Could you check a few things on this model? Use its own coordinates, in mm. A direction names the side the tool comes from. Give positions to 0.01 mm unless a question says otherwise; leave off trailing zeros. Loops run counter-clockwise (first coordinate to the right, second up) from the corner with the lowest first, then second, coordinate; pieces in that order, holes last.
1. Imagine slicing it at A-A (x = -54.5). List the corners of the cut face in (y, z) for me, plus the area to 3 significant figures.
2. For faces 4 (the cylindrical face through (-2.52, -3.79, -17.07)), 5 (the cylindrical face through (-52.874, -11.923, 3.755)), 6 (the flat face through (6.801, 13, -13)), 7 (the cylindrical face through (-34.37, -29.97, 1.32)), 8 (the conical face through (-12.821, -14.747, -11.307)), which set-ups out of +Z, -Z, +X, -X, +Y, -Y let a thin tool reach every point of the face, with its end or its side?
3. Imagine slicing it at B-B (y = -26). Count the separate pieces of the cut face and the enclosed holes in it, plus the area to 3 significant figures.
4. For P1, Ø8, axis at x = -2, y = 17, coming from the -Z side; P2, Ø5, axis at x = -44, z = -15, coming from the -Y side; P3, Ø1, axis at x = -39, y = 10, coming from the -Z side, each with a flat end and sliding along its axis, tell me the tip position at first contact or that it passes through.
5. I need wall thicknesses on line 1 along X through (y, z) = (-1, 26); line 2 along X through (y, z) = (-25, -13); line 3 along X through (y, z) = (11.5, 4). Which ranges of each line are inside material? Lowest first, please.
6. Thinking about a two-plate mould opening in Z: for faces 1 (the flat face through (-12.099, 0, 0)), 2 (the flat face through (-44, 0, -13)), 3 (the cylindrical face through (-10.72, -1.32, -29.97)), which applies, +Z half, -Z half, draft (parallel to the pull), parting line (faces both ways), or undercut?
7. Imagine slicing it at C-C (x = -31.5). List the corners of the cut face in (y, z) for me.
```python
from build123d import *

# Parameters (mm, degrees)
F2_R      = 17.485
F3_DEPTH  = 18.9
F6_R      = 30
F4_R      = 18
F8_DEPTH  = 19
F9_R      = 12.5
F10_DEPTH = 18


with BuildPart() as f1:
    # F0 (on Front) → F1 (revolve)
    with BuildSketch(Plane.XZ):
        with BuildLine():
            Line((-12.1993720531, 30), (-12.1993720531, 0))
            Line((-12.1993720531, 0), (6.8006279469, 0))
            Line((6.8006279469, 0), (6.8006279469, 30))
            Line((6.8006279469, 30), (3.8006279469, 30))
            add(Edge.make_bspline(
                [(-9.1993720531, 30), (-9.1993720531, 23.015), (-2.6993720531, 23.015), (3.8006279469, 23.015), (3.8006279469, 30)],
                knots=[4.7123889804, 4.7123889804, 4.7123889804, 6.2831853072, 6.2831853072, 7.853981634, 7.853981634, 7.853981634], degree=2, weights=[1, 0.7071067812, 1, 0.7071067812, 1]))
            Line((-9.1993720531, 30), (-12.1993720531, 30))
        make_face()
    revolve(axis=Axis((-2.6993720531, 0, 0), (1, 0, 0)))

    # F2 (on face) → F3 (cut)
    with BuildSketch(Plane.YZ.offset(6.8006279469)):
        Circle(F2_R)
    extrude(amount=-F3_DEPTH, mode=Mode.SUBTRACT)

    # F6 (on offset) → F7 section 0
    with BuildSketch(Plane.YZ.offset(-25)):
        Circle(F6_R)
    # F4 (on face) → F7 section 1
    with BuildSketch(Plane(origin=(-12.1993720531, 0, 0), x_dir=(0, -1, 0), z_dir=(-1, 0, 0))):
        Circle(F4_R)
    loft()

    # F8 (add): a face of the model
    f8_faces = [f1.faces().sort_by_distance(p)[0] for p in [
        (-25, 0, 0),
    ]]
    extrude(f8_faces, amount=F8_DEPTH)

    # F9 (on face) → F10 (join)
    with BuildSketch(Plane(origin=(-44, 0, 0), x_dir=(0, -1, 0), z_dir=(-1, 0, 0))):
        Circle(F9_R)
    extrude(amount=F10_DEPTH)


solid = f1.part
```
Derived:
1. outline: circle Ø25 at (0, 0)
1. area: 491 mm2
2. face 4: +X
2. face 5: -X
2. face 6: +Z, -Z, +X, +Y, -Y
2. face 7: +X, -X
2. face 8: none
3. separate pieces: 3
3. enclosed holes: 0
3. area: 868 mm2
4. P1: stops at z = -19.56
4. P2: stops at y = -27.27
4. P3: stops at z = -28.46
5. line 1: x = -44 to -20.75, -12.2 to -8.04, 2.64 to 6.8
5. line 2: x = -44 to -23.06, -12.2 to -8.97, 3.58 to 6.8
5. line 3: x = -62 to -12.1
6. face 1: undercut
6. face 2: draft
6. face 3: parting line
7. outline: circle Ø60 at (0, 0)
